from build123d import *

# Parameters (mm, degrees)
CYLINDER018_R        = 1.6
CYLINDER018_DEPTH    = 10
CYLINDER017_R        = 1.6
CYLINDER017_DEPTH    = 10
PAD_DEPTH            = 18
SKETCH002_R          = 0.75
PAD001_DEPTH         = 1.8
CYLINDER_R           = 5.025
CYLINDER_DEPTH       = 1.8
BODY_PLACEMENT_ANGLE = 60
CYLINDER006_R        = 4.95
CYLINDER006_DEPTH    = 14
EXTRUDE_DEPTH        = 4
CYLINDER005_R        = 4.95
CYLINDER005_DEPTH    = 14


with BuildPart() as cylinder018:
    # Cylinder018 → Cylinder018 (new body)
    with BuildSketch(Plane(origin=(-30, 0, -3), x_dir=(1, 0, 0), z_dir=(0, 0, 1))):
        Circle(CYLINDER018_R)
    extrude(amount=CYLINDER018_DEPTH)


with BuildPart() as fusion021:
    # Cylinder017 → Cylinder017 (new body)
    with BuildSketch(Plane.XY.offset(-3)):
        Circle(CYLINDER017_R)
    extrude(amount=CYLINDER017_DEPTH)

    # Fusion019: union Cylinder018
    add(cylinder018.part)


with BuildPart() as fusion021_1:
    # Fusion019 placement: moved
    add(fusion021.part.moved(Location((-18, 1, 0))))


with BuildPart() as motorbody:
    # Sketch001 → Pad (new body)
    with BuildSketch(Plane.XY):
        with BuildLine():
            ThreePointArc((-2.940238, 4.075), (-5.025, 0), (-2.940238, -4.075))
            Line((-2.940238, -4.075), (2.940238, -4.075))
            ThreePointArc((2.940238, -4.075), (5.025, 0), (2.940238, 4.075))
            Line((-2.940238, 4.075), (2.940238, 4.075))
        make_face()
    extrude(amount=PAD_DEPTH)

    # Sketch002 → Pad001 (join)
    with BuildSketch(Plane.XY):
        with BuildLine():
            ThreePointArc((1.85, 6.95), (0, 8.8), (-1.85, 6.95))
            Line((-1.85, 6.95), (-1.85, -6.950003))
            ThreePointArc((-1.85, -6.950003), (2e-06, -8.8), (1.85, -6.949999))
            Line((1.85, 6.95), (1.85, -6.949999))
        make_face()
        with Locations((0, 6.95)):
            Circle(SKETCH002_R, mode=Mode.SUBTRACT)
        with Locations((0, -6.95)):
            Circle(SKETCH002_R, mode=Mode.SUBTRACT)
    extrude(amount=PAD001_DEPTH)

    # Cylinder → Cylinder (join)
    with BuildSketch(Plane.XY):
        Circle(CYLINDER_R)
    extrude(amount=CYLINDER_DEPTH)


with BuildPart() as motorbody_1:
    # Body placement: moved
    add(motorbody.part.rotate(Axis((0, 0, 0), (0, 0, -1)), BODY_PLACEMENT_ANGLE))


with BuildPart() as cylinder006:
    # Cylinder006 → Cylinder006 (new body)
    with BuildSketch(Plane(origin=(-33.693581, 0, -14), x_dir=(1, 0, 0), z_dir=(0, 0, 1))):
        Circle(CYLINDER006_R)
    extrude(amount=CYLINDER006_DEPTH)


with BuildPart() as extrude_body:
    # Sketch009 → Extrude (new body)
    with BuildSketch(Plane.XY):
        with BuildLine():
            ThreePointArc((-68.158607, 8), (-75.158607, 1), (-68.158607, -6))
            Line((-68.158607, -6), (2, -6))
            ThreePointArc((2, -6), (9, 1), (2, 8))
            Line((-68.158607, 8), (2, 8))
        make_face()
    extrude(amount=EXTRUDE_DEPTH)


with BuildPart() as rightdriveskid:
    # Cylinder005 → Cylinder005 (new body)
    with BuildSketch(Plane(origin=(-67.3872, 0, -14), x_dir=(1, 0, 0), z_dir=(0, 0, 1))):
        Circle(CYLINDER005_R)
    extrude(amount=CYLINDER005_DEPTH)

    # Fusion005: union Cylinder006, Extrude body
    add(cylinder006.part)
    add(extrude_body.part)

    # Cut002: cut MotorBody
    add(motorbody_1.part, mode=Mode.SUBTRACT)

    # Cut011: cut Fusion021
    add(fusion021_1.part, mode=Mode.SUBTRACT)


with BuildPart() as leftdriveskid:
    # Part__Mirroring003: instance of RightDriveSkid
    add(rightdriveskid.part.mirror(Plane(origin=(0, 0, 0), x_dir=(0, 1, 0), z_dir=(0, 0, 1))))


solid = leftdriveskid.part
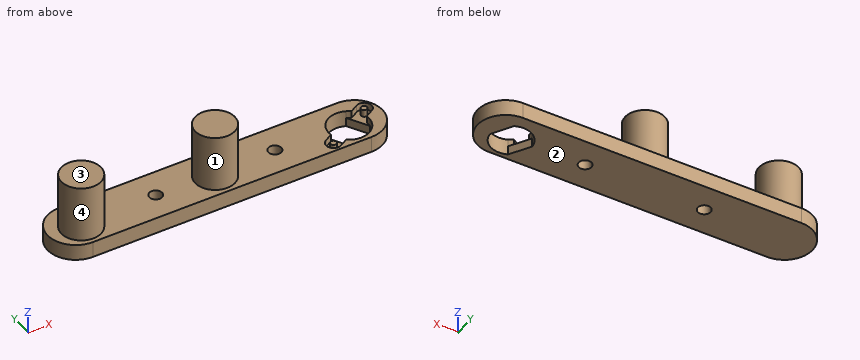
For this review, take the finished solid that the model builds, in its own axes (mm). Face numbers are marked on the shaded views. A direction names the side the tool comes from. Round coordinates to 2 decimals unless told otherwise and drop trailing zeros. Write each loop counter-clockwise with the first axis right and the second up, starting at its lowest first coordinate (ties: lowest second). Pieces come first, ordered by that corner, then holes. Notation, with made-up numbers: (46.5, 3) -> (81.5, 3) arc R5 ccw to (81.5, 8) -> close; hole circle Ø9 at (21, 42.25). An arc over 180 degrees is marked (long way). Use CSV: the item, a comma, the result in double quotes.
(1) Draft analysis for pull direction X (two halves, no side actions). For the marked faces 1 and 2, state which applies: +X half, -X half, draft (parallel to the pull), parting line (faces both ways), or undercut.
Computed values:
face 1,"undercut"
face 2,"draft"
(2) To check wall thickness, follow L1, parallel to X at y = 1, z = -2.1; L2, parallel to Y at x = -18, z = -0.85; L3, parallel to X at y = -0.25, z = 2.5. State the ranges of each line that lie inside material, in increasing order. Write a range as [from, to].
Computed values:
L1,"[-75.16, -49.6], [-46.4, -19.6], [-16.4, -4.92], [4.13, 9]"
L2,"[-6, -0.6], [2.6, 8]"
L3,"[-72.33, -62.44], [-38.64, -28.75]"
(3) Consider section A-A, the plane x = -18. Give the boundary of the cut face in (y, z).
Computed values:
outline,"(-6, -4) -> (-0.6, -4) -> (-0.6, 0) -> (-6, 0) -> close; (2.6, -4) -> (8, -4) -> (8, 0) -> (2.6, 0) -> close"
(4) Consider section C-C, the plane x = -34. Give the boundary of the cut face in (y, z).
Computed values:
outline,"(-6, -4) -> (8, -4) -> (8, 0) -> (4.94, 0) -> (4.94, 14) -> (-4.94, 14) -> (-4.94, 0) -> (-6, 0) -> close"
(5) Clearance check with flat-ended pins moving along their axes: P1, Ø1, axis at x = -61, z = 3.5, coming from the -Y side; P2, Ø1.6, axis at x = -6, y = -3.5, coming from the +Z side; P3, Ø8, axis at x = -64.5, z = 1.5, coming from the -Y side; P4, Ø8, axis at x = -33.5, z = 11, coming from the +Y side. State where each tip first meets the part, or that it passes through.
Computed values:
P1,"through"
P2,"z = 0"
P3,"y = -6"
P4,"y = 4.95"
(6) For the marked faces 3 and 4, list the 3-axis set-ups (+Z, -Z, +X, -X, +Y, -Y) from which the entire face can be reached by the end or side of a thin tool; tool diameter is ignored.
Computed values:
face 3,"+Z, +X, -X, +Y, -Y"
face 4,"+Z"
(7) Consider section B-B, the plane z = 6.75. Give the boundary of the cut face in (x, y).
Computed values:
outline,"circle Ø9.9 at (-67.39, 0); circle Ø9.9 at (-33.69, 0)"
